The listing builds one solid part. Answer for the finished solid, in the listing's coordinates (mm). A direction names the side the tool comes from. Give positions to 0.01 mm unless a question says otherwise; leave off trailing zeros. Order: outer loops, then holes, each group sorted by start corner. A loop starts at its lowest first (then second) coordinate and runs counter-clockwise, first axis right, second up. Notation, with made-up numbers: (22.5, 2) - (48.5, 2) arc R28 ccw to (48.5, 35) - close; hole circle Ø3 at (85.25, 41). An arc over 180 degrees is marked (long way). Answer in a Markdown table with one row per item. Add a question column.
```python
from build123d import *

# Parameters (mm, degrees)
CROQUIS1_W                                           = 20
CROQUIS1_H                                           = 20
SALIENTE_EXTRUIR1_DEPTH                              = 10
PERFORADOR_PARA_ROSCAR_PARA_MACHO_DE_ROS_D           = 5
REFRENTADO_PARA_TORNILLO_TAP_N_CON_CABEZ_D           = 3.4
REFRENTADO_PARA_TORNILLO_TAP_N_CON_CABEZ_CSINK_D     = 5
REFRENTADO_PARA_TORNILLO_TAP_N_CON_CABEZ_CSINK_ANGLE = 90
TALADRO_DE_MARGEN_PARA_M31_D                         = 3.4
CROQUIS17_R                                          = 3.1
CORTAR_EXTRUIR1_DEPTH                                = 20
TALADRO_DE_MARGEN_PARA_M32_D                         = 3.4
TALADRO_DE_MARGEN_PARA_M32_DEPTH                     = 7
CROQUIS21_R                                          = 0.9
CORTAR_EXTRUIR2_DEPTH                                = 2.75


with BuildPart() as part:
    # Croquis1 → Saliente-Extruir1 (new body)
    with BuildSketch(Plane(origin=(0, 0, 0), x_dir=(1, 0, 0), z_dir=(0, 1, 0))):
        Rectangle(CROQUIS1_W, CROQUIS1_H)
    extrude(amount=SALIENTE_EXTRUIR1_DEPTH)

    # Perforador para roscar para macho de roscar para M6x1.01 (through all)
    with Locations(Plane(origin=(0, 10, 0), x_dir=(1, 0, 0), z_dir=(0, 1, 0))):
        with Locations((0, -3.5)):
            Hole(PERFORADOR_PARA_ROSCAR_PARA_MACHO_DE_ROS_D / 2)

    # Refrentado para tornillo tapón con cabeza plana de clavija de M31 (through all)
    with Locations(Plane(origin=(0, 10, 0), x_dir=(1, 0, 0), z_dir=(0, 1, 0))):
        with Locations((-7, -5), (7, -5)):
            CounterSinkHole(REFRENTADO_PARA_TORNILLO_TAP_N_CON_CABEZ_D / 2, REFRENTADO_PARA_TORNILLO_TAP_N_CON_CABEZ_CSINK_D / 2, counter_sink_angle=REFRENTADO_PARA_TORNILLO_TAP_N_CON_CABEZ_CSINK_ANGLE)

    # Taladro de margen para M31 (through all)
    with Locations(Plane(origin=(0, 10, 0), x_dir=(1, 0, 0), z_dir=(0, 1, 0))):
        with Locations((0, 6)):
            Hole(TALADRO_DE_MARGEN_PARA_M31_D / 2)

    # Croquis17 → Cortar-Extruir1 (cut)
    with BuildSketch(Plane(origin=(10, 0, 0), x_dir=(0, 0, -1), z_dir=(1, 0, 0))):
        with Locations((5.5, 5)):
            Circle(CROQUIS17_R)
    extrude(amount=-CORTAR_EXTRUIR1_DEPTH, mode=Mode.SUBTRACT)

    # Taladro de margen para M32
    with Locations(Plane(origin=(10, 0, 0), x_dir=(0, 0, 1), z_dir=(1, 0, 0))):
        with Locations((0, -5)):
            Hole(TALADRO_DE_MARGEN_PARA_M32_D / 2, depth=TALADRO_DE_MARGEN_PARA_M32_DEPTH)

    # Croquis21 → Cortar-Extruir2 (cut)
    with BuildSketch(Plane.ZY.offset(-10)):
        with Locations((-1.5, 7.75)):
            Circle(CROQUIS21_R)
    extrude(amount=CORTAR_EXTRUIR2_DEPTH, mode=Mode.SUBTRACT)


solid = part.part
```
(1) Straight lines are drawn through the part: line 1 (Z direction, x = 0, y = 6.25); line 2 (Z direction, x = 0, y = 6.75); line 3 (X direction, y = 7, z = 5). For each, find the intervals that lie inside material, in ascending order.
(2) The mould has two halves that part along Z. Classify faces 3 (the face through (-1.34, 4.93, 1.39)), 4 (the face through (0, 5, -10)), 5 (the face through (0, 0, 0)): +Z half, -Z half, draft (parallel to the pull), parting line (faces both ways), or undercut.
(3) For faces 1 (the face through (7.25, 8, -2)), 2 (the face through (10, 5, 2)), determine the directions among +Z, -Z, +X, -X, +Y, -Y from which every point of the face is accessible in a straight line to the end or side of a thin tool.
(4) Find section D-D, the plane y = 9.75. Write down the section's boundary in (x, z).
(5) Each of these flat-tipped pins is pushed along its axis until it touches: P1, Ø1.7, axis at y = 5, z = 0, coming from the +X side; P2, Ø8, axis at x = -2.5, z = -0.5, coming from the -Y side; P3, Ø3, axis at x = 7, z = 5, coming from the -Y side. Where does it stop, or does it pass through?
(6) Find section C-C, the plane z = -3. Write down the section's boundary in (x, y).
(7) Find section B-B, the plane x = -7. Write down the section's boundary in (y, z).
(8) Find section A-A, the plane y = 5. Write down the section's boundary in (x, z).
Answer key:
| question | item | result |
|---|---|---|
| 1 | line 1 | -10 to -8.34, -2.66 to 1, 6 to 10 |
| 1 | line 2 | -10 to -8.06, -2.94 to 1, 6 to 10 |
| 1 | line 3 | -10 to -8.7, -5.3 to -2, 2 to 5.3, 8.7 to 10 |
| 2 | face 3 | undercut |
| 2 | face 4 | -Z half |
| 2 | face 5 | draft |
| 3 | face 1 | +X |
| 3 | face 2 | +Z, -Z, +X, +Y, -Y |
| 4 | outline | (-10, -10) - (10, -10) - (10, 10) - (-10, 10) - close; hole circle Ø4.5 at (-7, 5); hole circle Ø5 at (0, 3.5); hole circle Ø3.4 at (0, -6); hole circle Ø4.5 at (7, 5) |
| 5 | P1 | x = 3 |
| 5 | P2 | y = 0 |
| 5 | P3 | through |
| 6 | outline | (-10, 0) - (10, 0) - (10, 3.17) - (-10, 3.17) - close; (-10, 6.83) - (10, 6.83) - (10, 10) - (-10, 10) - close |
| 7 | outline | (0, -10) - (10, -10) - (10, 2.5) - (9.2, 3.3) - (0, 3.3) - close; (0, 6.7) - (9.2, 6.7) - (10, 7.5) - (10, 10) - (0, 10) - close; hole circle Ø6.2 at (5, -5.5) |
| 8 | outline | (-10, -10) - (10, -10) - (10, -8.6) - (-10, -8.6) - close; (-10, -2.4) - (10, -2.4) - (10, -1.7) - (3, -1.7) - (3, 1.7) - (10, 1.7) - (10, 10) - (-10, 10) - close; hole circle Ø3.4 at (-7, 5); hole circle Ø5 at (0, 3.5); hole circle Ø3.4 at (7, 5) |
